```python
from build123d import *

# Parameters (mm, degrees)
SKETCH1_W           = 38.1
SKETCH1_H           = 11.1252
SKETCH1_R           = 2.5
SKETCH1_W_2         = 11.1252
SKETCH1_H_2         = 38.1
BOSS_EXTRUDE1_DEPTH = 22.2504
FILLET1_R           = 3
FILLET2_R           = 1.5


with BuildPart() as part:
    # Sketch1 → Boss-Extrude1 (new body)
    # profile 1 of 3: a face of its own
    with BuildSketch(Plane(origin=(0, 0, 0), x_dir=(1, 0, 0), z_dir=(0, 1, 0))):
        with Locations((19.05, -5.5626)):
            Rectangle(SKETCH1_W, SKETCH1_H)
        with Locations(Location((6.35, -4.7752, 0), (0, 0, 90))):
            Circle(SKETCH1_R, mode=Mode.SUBTRACT)
        with Locations(Location((31.75, -4.7752, 0), (0, 0, 90))):
            Circle(SKETCH1_R, mode=Mode.SUBTRACT)
    # profile 2 of 3: a face of its own
    with BuildSketch(Plane(origin=(0, 0, 0), x_dir=(1, 0, 0), z_dir=(0, 1, 0))):
        Polygon((100.0252, -29.649448268), (100.0252, -36.5252), (88.9, -36.5252), (38.1, -11.1252), (38.1, 0), (40.726303463, 0), align=None)
    # profile 3 of 3: a face of its own
    with BuildSketch(Plane(origin=(0, 0, 0), x_dir=(1, 0, 0), z_dir=(0, 1, 0))):
        with Locations((94.4626, -55.5752)):
            Rectangle(SKETCH1_W_2, SKETCH1_H_2)
        with Locations(Location((95.25, -68.2752, 0), (0, 0, 90))):
            Circle(SKETCH1_R, mode=Mode.SUBTRACT)
        with Locations(Location((95.25, -42.8752, 0), (0, 0, 90))):
            Circle(SKETCH1_R, mode=Mode.SUBTRACT)
    extrude(amount=BOSS_EXTRUDE1_DEPTH)

    # Fillet1
    fillet1_edges = [part.edges().sort_by_distance(p)[0] for p in [
        (0, 11.1252, 11.1252),
        (0, 11.1252, 0),
        (40.726303463, 11.1252, 0),
        (100.0252, 11.1252, 29.649448268),
        (100.0252, 11.1252, 74.6252),
        (88.9, 11.1252, 74.6252),
        (88.9, 11.1252, 36.5252),
        (38.1, 11.1252, 11.1252),
    ]]
    fillet(fillet1_edges, radius=FILLET1_R)

    # Fillet2
    fillet2_edges = [part.edges().sort_by_distance(p)[0] for p in [
        (21.509049765, 0, 0),
        (21.509049765, 22.2504, 0),
        (20.195898034, 0, 11.1252),
        (0, 0, 5.5626),
        (69.863290552, 0, 14.568493544),
        (100.0252, 0, 51.564375117),
        (94.4626, 0, 74.6252),
        (88.9, 0, 55.002250983),
        (62.98753882, 0, 23.56896941),
        (0.878679656, 0, 0.878679656),
        (0.878679656, 0, 10.246520344),
        (89.778679656, 0, 73.746520344),
        (99.146520344, 0, 73.746520344),
        (99.577152425, 0, 29.926356898),
        (40.707358292, 0, 0.080253032),
        (69.863290552, 22.2504, 14.568493544),
        (20.195898034, 22.2504, 11.1252),
        (62.98753882, 22.2504, 23.56896941),
        (88.9, 22.2504, 55.002250983),
        (94.4626, 22.2504, 74.6252),
        (100.0252, 22.2504, 51.564375117),
        (0, 22.2504, 5.5626),
        (0.878679656, 22.2504, 0.878679656),
        (0.878679656, 22.2504, 10.246520344),
        (89.778679656, 22.2504, 73.746520344),
        (99.146520344, 22.2504, 73.746520344),
        (99.577152425, 22.2504, 29.926356898),
        (40.707358292, 22.2504, 0.080253032),
        (38.081054829, 0, 11.205453032),
        (38.081054829, 22.2504, 11.205453032),
        (88.451952425, 0, 36.80210863),
        (88.451952425, 22.2504, 36.80210863),
    ]]
    fillet(fillet2_edges, radius=FILLET2_R)


solid = part.part
```
Design review of the part built by this model. Coordinates are the model's own, in mm. A direction names the side the tool comes from. Round coordinates to 2 decimals unless told otherwise and drop trailing zeros. Write each loop counter-clockwise with the first axis right and the second up, starting at its lowest first coordinate (ties: lowest second). Pieces come first, ordered by that corner, then holes.
Item 1: We need section C-C on y = 19.25. Write out the cut boundary in (x, z).
Item 2: We need section A-A on x = 6.35. Write out the cut boundary in (y, z), and give its area (3 significant figures).
Item 3: We need section B-B on z = 67. Write out the cut boundary in (x, y), and give its area (3 significant figures).
Item 4: Clearance check with flat-ended pins moving along their axes: pin 1 Ø9.5 at (y, z) = (11, 51) entering from -X; pin 2 Ø3 at (x, z) = (95.25, 68.28) entering from +Y; pin 3 Ø6 at (x, y) = (73.5, 8.5) entering from -Z; pin 4 Ø8 at (x, y) = (65, 5.5) entering from -Z. State where each tip first meets the part, or that it passes through.
Item 5: For probe 1 along Z at (x, y) = (31.75, 14); probe 2 along Z at (x, y) = (93, 9.75); probe 3 along X at (y, z) = (10, 56), list the stretches that pass through material, from the lowest coordinate up.
Item 6: The part is to be moulded in two halves that separate along X. For faces 3 (the flat face through (20, 11, 11.125)), 4 (the cylindrical face through (29.27, 10.97, 5.1)), 5 (the cylindrical face through (0.86, 11.26, 0.9)), 6 (the flat face through (69.464, 10.99, 14.369)), say which applies: +X half, -X half, draft (parallel to the pull), parting line (faces both ways), or undercut.
Item 7: We need section D-D on z = 56. Write out the cut boundary in (x, y).
Item 8: For faces 1 (the flat face through (0, 11, 6)), 2 (the flat face through (88.9, 11, 55)), list the 3-axis set-ups (+Z, -Z, +X, -X, +Y, -Y) from which the entire face can be reached by the end or side of a thin tool; tool diameter is ignored.
Returned:
1. outline: (0, 3) arc R3 ccw to (3, 0) - (40.02, 0) arc R3 ccw to (41.36, 0.32) - (98.37, 28.82) arc R3 ccw to (100.03, 31.5) - (100.03, 71.63) arc R3 ccw to (97.03, 74.63) - (91.9, 74.63) arc R3 ccw to (88.9, 71.63) - (88.9, 38.38) arc R3 cw to (87.24, 35.7) - (38.73, 11.44) arc R3 cw to (37.39, 11.13) - (3, 11.13) arc R3 ccw to (0, 8.13) - close; hole circle Ø5 at (6.35, 4.78); hole circle Ø5 at (31.75, 4.78); hole circle Ø5 at (95.25, 42.88); hole circle Ø5 at (95.25, 68.28)
2. outline: (0, 1.5) arc R1.5 ccw to (1.5, 0) - (20.75, 0) arc R1.5 ccw to (22.25, 1.5) - (22.25, 2.28) - (0, 2.28) - close; (0, 7.28) - (22.25, 7.28) - (22.25, 9.63) arc R1.5 ccw to (20.75, 11.13) - (1.5, 11.13) arc R1.5 ccw to (0, 9.63) - close
2. area: 134 mm2
3. outline: (88.9, 1.5) arc R1.5 ccw to (90.4, 0) - (93.1, 0) - (93.1, 22.25) - (90.4, 22.25) arc R1.5 ccw to (88.9, 20.75) - close; (97.4, 0) - (98.53, 0) arc R1.5 ccw to (100.03, 1.5) - (100.03, 20.75) arc R1.5 ccw to (98.53, 22.25) - (97.4, 22.25) - close
3. area: 150 mm2
4. pin 1: stops at x = 88.9
4. pin 2: passes through
4. pin 3: stops at z = 14.89
4. pin 4: stops at z = 10.14
5. probe 1: z = 0 to 2.28, 7.28 to 11.13
5. probe 2: z = 26.14 to 41.79, 43.96 to 67.19, 69.36 to 74.63
5. probe 3: x = 88.9 to 100.03
6. face 3: draft
6. face 4: undercut
6. face 5: -X half
6. face 6: +X half
7. outline: (88.9, 1.5) arc R1.5 ccw to (90.4, 0) - (98.53, 0) arc R1.5 ccw to (100.03, 1.5) - (100.03, 20.75) arc R1.5 ccw to (98.53, 22.25) - (90.4, 22.25) arc R1.5 ccw to (88.9, 20.75) - close
8. face 1: +Z, -Z, -X, +Y, -Y
8. face 2: +Z, -X, +Y, -Y
